For this review, take the finished solid that the model builds, in its own axes (mm). A direction names the side the tool comes from. Round coordinates to 2 decimals unless told otherwise and drop trailing zeros. Write each loop counter-clockwise with the first axis right and the second up, starting at its lowest first coordinate (ties: lowest second). Pieces come first, ordered by that corner, then holes. Notation, with made-up numbers: (-27.75, -19.75) -> (-6.75, -19.75) arc R12 ccw to (-6.75, -11.75) -> close; hole circle Ø5 at (-0.5, 79.25). An arc over 180 degrees is marked (long way). Answer in a Markdown table with one row per item.
from build123d import *

# Parameters (mm, degrees)
F0_R            = 14.75
F2_DEPTH        = 7
F3_R            = 19.75
F3_R_2          = 14.75
F4_DEPTH        = 5
F6_D            = 5.5
F6_CSINK_D      = 11.2
F6_CSINK_ANGLE  = 90
F6_COPIES_COUNT = 3
F7_SIZE         = 1


# Not quite as in the source:
# - a pattern or mirror of a feature is missing from the dataset's text; its kind, count and spacing are read off the source's solid


with BuildPart() as f2:
    # F0 (on Top) → F2 (new body)
    with BuildSketch(Plane.XY):
        Circle(F0_R)
    extrude(amount=-F2_DEPTH)

    # F3 (on face) → F4 (join)
    with BuildSketch(Plane.XY):
        Circle(F3_R)
        Circle(F3_R_2, mode=Mode.SUBTRACT)
        Circle(F3_R_2)
    extrude(amount=F4_DEPTH)

    # F6 (through all)
    with Locations(Plane.XY.offset(5)):
        with Locations((-10, 0)):
            f6 = CounterSinkHole(F6_D / 2, F6_CSINK_D / 2, counter_sink_angle=F6_CSINK_ANGLE)

    # F6_copies: F6 ×3 about axis
    f6_copies_axis = Axis((0, 0, 0), (0, 0, 1))
    for i in range(1, F6_COPIES_COUNT):
        add(f6.rotate(f6_copies_axis, i * 360 / F6_COPIES_COUNT), mode=Mode.SUBTRACT)

    # F7
    f7_edges = [f2.edges().sort_by_distance(p)[0] for p in [
        (-19.75, 0, 5),
        (-19.75, 0, 0),
    ]]
    chamfer(f7_edges, length=F7_SIZE)


solid = f2.part
1) Clearance check with flat-ended pins moving along their axes: pin 1 Ø6 at (y, z) = (-6.5, -2) entering from -X; pin 2 Ø5 at (x, z) = (-0.5, 1) entering from +Y; pin 3 Ø9 at (x, y) = (5, -8.66) entering from +Z. State where each tip first meets the part, or that it passes through.
Solved:
| item | result |
|---|---|
| pin 1 | x = -18.8 |
| pin 2 | y = 19.75 |
| pin 3 | z = 3.9 |
2) For line 1 (Y direction, x = 6.5, z = -0.75); line 2 (Y direction, x = 5, z = -1); line 3 (Y direction, x = -10, z = -1.75), list the stretches that pass through material, from the lowest coordinate up. Write a range as [from, to].
Solved:
| item | result |
|---|---|
| line 1 | [-13.24, -10.97], [-6.36, 6.36], [10.97, 13.24] |
| line 2 | [-13.88, -11.41], [-5.91, 5.91], [11.41, 13.88] |
| line 3 | [-10.84, -2.75], [2.75, 10.84] |
3) Mouldability with a two-part tool opening along Y and no side actions: class faces 1 (the cylindrical face through (14.07, 4.43, -3.45)), 2 (the conical face through (-9.624, 2.864, 2.288)), 3 (the flat face through (0, 0, 5)), 4 (the cylindrical face through (-12.54, -1.05, -2.49)) as pulls with the +Y half, pulls with the -Y half, needs draft (parallel to the pull), parting line crosses it, or undercut.
Solved:
| item | result |
|---|---|
| face 1 | parting line crosses it |
| face 2 | undercut |
| face 3 | needs draft |
| face 4 | undercut |
4) Consider section A-A on y = 0. State the section outline as (x, z) points, then the cut area to 3 significant figures.
Solved:
| item | result |
|---|---|
| outline | (-19.75, 1) -> (-18.75, 0) -> (-14.75, 0) -> (-14.75, -7) -> (-12.75, -7) -> (-12.75, 2.15) -> (-15.6, 5) -> (-18.75, 5) -> (-19.75, 4) -> close; (-7.25, -7) -> (14.75, -7) -> (14.75, 0) -> (18.75, 0) -> (19.75, 1) -> (19.75, 4) -> (18.75, 5) -> (-4.4, 5) -> (-7.25, 2.15) -> close |
| area | 328 mm² |
5) For faces 5 (the flat face through (8.25, -12.41, 0)), 6 (the cylindrical face through (-14.6, 13.3, 2.5)), list the 3-axis set-ups (+Z, -Z, +X, -X, +Y, -Y) from which the entire face can be reached by the end or side of a thin tool; tool diameter is ignored.
Solved:
| item | result |
|---|---|
| face 5 | -Z |
| face 6 | +Z, -Z |
6) Consider section B-B on x = 3.5. State how many separate pieces and enclosed holes the cut face has, then the cut area to 3 significant figures.
Solved:
| item | result |
|---|---|
| separate pieces | 3 |
| enclosed holes | 0 |
| area | 264 mm² |
7) Consider section C-C on z = -1. State the section outline as (x, y) points (3 decimals).
Solved:
| item | result |
|---|---|
| outline | circle Ø29.5 at (0, 0); hole circle Ø5.5 at (-10, 0); hole circle Ø5.5 at (5, -8.66); hole circle Ø5.5 at (5, 8.66) |
